from build123d import *

# Parameters (mm, degrees)
F0_R     = 15.875
F1_DEPTH = 76.2
F3_DEPTH = 25.4
F4_DEPTH = 25.4


with BuildPart() as f1:
    # F0 (on Top) → F1 (new body)
    with BuildSketch(Plane.XY):
        Circle(F0_R)
    extrude(amount=F1_DEPTH)

    # F2 (on Right) → F3 (join)
    with BuildSketch(Plane.YZ):
        with BuildLine():
            Line((50.8, 0), (0, 0))
            Line((0, 0), (-50.8, 0))
            ThreePointArc((-50.8, 0), (0, -19.117184), (50.8, 0))
        make_face()
    extrude(amount=F3_DEPTH)

    # F2 (on Right) → F4 (join)
    with BuildSketch(Plane.YZ):
        with BuildLine():
            Line((50.8, 0), (0, 0))
            Line((0, 0), (-50.8, 0))
            ThreePointArc((-50.8, 0), (0, -19.117184), (50.8, 0))
        make_face()
    extrude(amount=-F4_DEPTH)


solid = f1.part
Model file for the job. Use its own axes, mm. A direction names the side the tool comes from. Round coordinates to 2 decimals unless told otherwise and drop trailing zeros. Loops run counter-clockwise (first coordinate to the right, second up) from the corner with the lowest first, then second, coordinate; pieces in that order, holes last.
1. Wall check: probe 1 along Z at (x, y) = (17, -34.5); probe 2 along Z at (x, y) = (12, -10); probe 3 along Y at (x, z) = (9.5, -9.5). Give the ranges that are in metal, low to high.
Check values:
probe 1: z = -10.96 to 0
probe 2: z = -18.47 to 76.2
probe 3: y = -37.28 to 37.28
2. Drop flat-ended pins along their axis: P1, Ø6, axis at y = 32, z = 3.5, coming from the -X side; P2, Ø10, axis at x = 4.5, y = 15, coming from the -Z side; P3, Ø12, axis at y = -20, z = 21.5, coming from the +X side; P4, Ø1, axis at y = -12, z = 19.5, coming from the +X side. Give the stop position or say it passes through.
Check values:
P1: passes through
P2: stops at z = -18.47
P3: stops at x = 7.48
P4: stops at x = 10.94
3. Band-saw the part on D-D, the plane x = 22.5. List the corners of the cut face in (y, z), and give its area (3 significant figures).
Check values:
outline: (-50.8, 0) arc R77.05 ccw to (50.8, 0) - close
area: 1,330 mm2
4. Band-saw the part on A-A, the plane y = 0. List the corners of the cut face in (x, z) (3 decimals), and give its area (3 significant figures).
Check values:
outline: (-25.4, -19.117) - (25.4, -19.117) - (25.4, 0) - (15.875, 0) - (15.875, 76.2) - (-15.875, 76.2) - (-15.875, 0) - (-25.4, 0) - close
area: 3,390 mm2
5. Band-saw the part on B-B, the plane x = 0. List the corners of the cut face in (y, z) (3 decimals).
Check values:
outline: (-50.8, 0) arc R77.054 ccw to (50.8, 0) - (15.875, 0) - (15.875, 76.2) - (-15.875, 76.2) - (-15.875, 0) - close
6. Band-saw the part on C-C, the plane z = 55. List the corners of the cut face in (x, y) (3 decimals).
Check values:
outline: circle Ø31.75 at (0, 0)
7. Tool access for faces 1 (the cylindrical face through (-3.441, -15.497, 37.567)), 2 (the flat face through (25.4, -1, -7)): list every direction of +Z, -Z, +X, -X, +Y, -Y with a clear straight run to the whole face (end or side of a thin tool).
Check values:
face 1: +Z
face 2: +Z, -Z, +X, +Y, -Y
